Read the model definition and answer for the solid it produces. Units are mm, in the model's axes. Face numbers are marked on the shaded views. A direction names the side the tool comes from. Coordinates: 2 decimals unless noted, no trailing zeros. Loops run counter-clockwise (first coordinate to the right, second up) from the corner with the lowest first, then second, coordinate; pieces in that order, holes last. Notation, with made-up numbers: (61, 46) -> (98, 46) arc R21 cw to (98, 80) -> close; hole circle Ø5 at (47.5, 40.5). An arc over 180 degrees is marked (long way). Answer as a JSON object with one key per item and string values. Group by question number.
1) Which of the six approach directions +Z, -Z, +X, -X, +Y, -Y give full straight-line access (tool end or side, diameter ignored) to the marked faces 4, 5, 6, 7 and 8?
2) Section A-A, the plane x = 0 is taken. Give the vertices of the cut face in (y, z), plus the area to 3 significant figures.
3) Determine the mould class of the marked faces 1, 2 and 3 for opening direction X: released by +X, released by -X, zero draft, split by the parting line, or undercut.
4) Consider probe 1 along X at (y, z) = (-7.4, 8.5); probe 2 along Z at (x, y) = (0, -6.85); probe 3 along Z at (x, y) = (-1, -4.75). Determine where each line is inside the solid, lowest interval first. Write a range as [from, to].
5) Section C-C, the plane z = -8.5 is taken. Give the vertices of the cut face in (x, y), plus the area to 3 significant figures.
6) Section B-B, the plane y = -4.75 is taken. Give the vertices of the cut face in (x, z), plus the area to 3 significant figures.
7) Flat-ended cylindrical pins translate along their axes: P1, Ø4, axis at x = 1, z = -7.5, coming from the +Y side; P2, Ø1.5, axis at x = -0.5, y = -4.5, coming from the +Z side; P3, Ø2, axis at x = 0, z = 1, coming from the -Y side. Find the tip coordinate at first contact, or state that the pin passes through.
8) Section D-D, the plane x = -1 is taken. Give the vertices of the cut face in (y, z), plus the area to 3 significant figures.
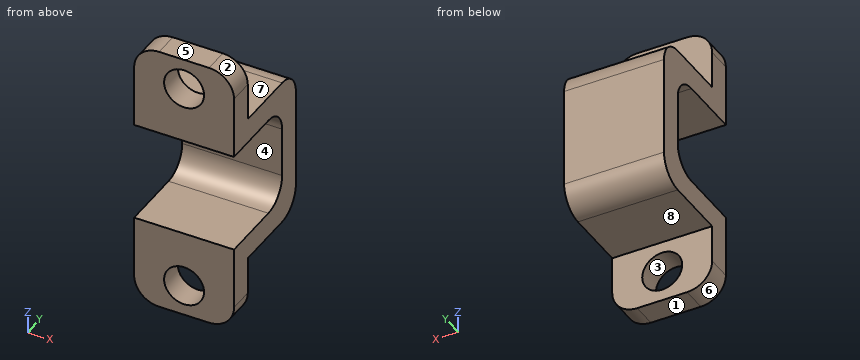
Autodesk Inventor part; units mm, degrees
ref_plane "YZ Plane" through (0, 0, 0) normal (1, 0, 0) x (0, 1, 0)
ref_plane "XZ Plane" through (0, 0, 0) normal (0, 1, 0) x (-1, 0, 0)
ref_plane "XY Plane" through (0, 0, 0) normal (0, 0, 1) x (1, 0, 0)
sketch "Skizze1" plane through (0, 0, 0) normal (0, 1, 0) x (-1, 0, 0)
  line L0 (4, -6) -> (-4, -6)
  line L1 (-4, -6) -> (-4, 6)
  line L2 (-4, 6) -> (4, 6)
  line L3 (4, 6) -> (4, -6)
  line L4 (0, -8.4) -> (0, 8.4)
  line L5 (-5.6, 0) -> (5.6, 0)
  point P0 (0, 0)
  dimension "d0" = 8
  dimension "d1" = 12
extrude "Extrusion1" add sketch "Skizze1" along normal mid plane 2
sketch "Skizze2" plane through (0, -1, 0) normal (0, -1, 0) x (1, 0, 0)
  line L0 (-4, -6) -> (-4, 6)
  line L1 (4, 6) -> (4, -6)
  line L2 (-4, -6) -> (4, -6)
  line L3 (4, -6) -> (4, -4)
  line L4 (4, -4) -> (-4, -4)
  line L5 (-4, -4) -> (-4, -6)
  line L6 (-4, 6) -> (4, 6)
  line L7 (4, 6) -> (4, 4)
  line L8 (4, 4) -> (-4, 4)
  line L9 (-4, 4) -> (-4, 6)
  point P0 (0, 0)
  dimension "d4" = 2
  dimension "d5" = 2
extrude "Extrusion2" add sketch "Skizze2" along normal blind 7 contours L0 L4 L1 L2 | L0 L6 L1 L8
sketch "Skizze3" plane through (4, 1, 6) normal (1, 0, 0) x (0, 0, -1)
  line L0 (2, -9) -> (0, -9)
  line L1 (0, -9) -> (-5, -9)
  line L2 (-5, -9) -> (-5, -7)
  line L3 (-5, -7) -> (0, -7)
  line L4 (0, -7) -> (0, -9)
  line L5 (12, -9) -> (10, -9)
  line L6 (12, -9) -> (17, -9)
  line L7 (17, -9) -> (17, -7)
  line L8 (17, -7) -> (12, -7)
  line L9 (12, -7) -> (12, -9)
  point P0 (6, -1)
  dimension "d8" = 5
  dimension "d9" = 2
  dimension "d10" = 5
  dimension "d11" = 2
extrude "Extrusion3" add sketch "Skizze3" against normal blind 8
sketch "Skizze4" plane through (4, -6, 11) normal (0, 1, 0) x (1, 0, 0)
  circle A0 centre (-4, 2.5) radius 1.6
  line L0 (0, 5) -> (0, 0)
  line L1 (0, 0) -> (-8, 0)
  circle A1 centre (-4, 19.5) radius 1.6
  line L2 (0, 22) -> (0, 17)
  line L3 (0, 22) -> (-8, 22)
  point P0 (-4, 11)
  dimension "d14" = 3.2
  dimension "d15" = 4
  dimension "d16" = 2.5
  dimension "d17" = 3.2
  dimension "d18" = 4
  dimension "d19" = 2.5
extrude "Extrusion4" cut sketch "Skizze4" against normal up to surface (2 mm away)
fillet "Rundung1" radius 2 8 edges at (0, 1, 6) (0, 1, -6) (0, -1, 4) (0, -1, -4) (-4, -7, 11) (4, -7, 11) (4, -7, -11) (-4, -7, -11)
properties part number "Kabelhalterung"
Determined:
{
 "1": {"face 4": "+X, -X, -Y", "face 5": "+Z, +X, -X, +Y, -Y", "face 6": "-Z, -X, +Y, -Y", "face 7": "+Z, +X, -X, +Y", "face 8": "-Z, +X, -X, +Y"},
 "2": {"outline": "(-8, -11) -> (-6, -11) -> (-6, -10.1) -> (-8, -10.1) -> close; (-8, -6.9) -> (-6, -6.9) -> (-6, -6) -> (-1, -6) arc R2 ccw to (1, -4) -> (1, 4) arc R2 ccw to (-1, 6) -> (-6, 6) -> (-6, 6.9) -> (-8, 6.9) -> (-8, 4) -> (-3, 4) arc R2 cw to (-1, 2) -> (-1, -2) arc R2 cw to (-3, -4) -> (-8, -4) -> close; (-8, 10.1) -> (-6, 10.1) -> (-6, 11) -> (-8, 11) -> close", "area": "59.2 mm²"},
 "3": {"face 1": "zero draft", "face 2": "released by +X", "face 3": "undercut"},
 "4": {"probe 1": "[-4, -1.6], [1.6, 4]", "probe 2": "[-11, -10.1], [-6.9, -4], [4, 6.9], [10.1, 11]", "probe 3": "[-6, -4], [4, 6]"},
 "5": {"outline": "(-4, -8) -> (-1.6, -8) -> (-1.6, -6) -> (-4, -6) -> close; (1.6, -8) -> (4, -8) -> (4, -6) -> (1.6, -6) -> close", "area": "9.60 mm²"},
 "6": {"outline": "(-4, -6) -> (4, -6) -> (4, -4) -> (-4, -4) -> close; (-4, 4) -> (4, 4) -> (4, 6) -> (-4, 6) -> close", "area": "32.0 mm²"},
 "7": {"P1": "y = 0.32", "P2": "z = 6", "P3": "y = -1"},
 "8": {"outline": "(-8, -11) -> (-6, -11) -> (-6, -9.75) -> (-8, -9.75) -> close; (-8, -7.25) -> (-6, -7.25) -> (-6, -6) -> (-1, -6) arc R2 ccw to (1, -4) -> (1, 4) arc R2 ccw to (-1, 6) -> (-6, 6) -> (-6, 7.25) -> (-8, 7.25) -> (-8, 4) -> (-3, 4) arc R2 cw to (-1, 2) -> (-1, -2) arc R2 cw to (-3, -4) -> (-8, -4) -> close; (-8, 9.75) -> (-6, 9.75) -> (-6, 11) -> (-8, 11) -> close", "area": "62.0 mm²"}
}
